from build123d import *

# Parameters (mm, degrees)
SKETCH1_W          = 34
SKETCH1_H          = 25
EXTRUDE1_DEPTH     = 30
SKETCH2_W          = 34
SKETCH2_H          = 25
EXTRUDE2_DEPTH     = 5
CHAMFER1_SIZE      = 5
SKETCH3_R          = 1.75
CUT_EXTRUDE1_DEPTH = 47.717707411


with BuildPart() as part:
    # Sketch1 → Extrude1 (new body)
    with BuildSketch(Plane.XY):
        with Locations((-8.642624393, 54.051188485)):
            Rectangle(SKETCH1_W, SKETCH1_H)
    extrude(amount=-EXTRUDE1_DEPTH)

    # Sketch2 → Extrude2 (add)
    with BuildSketch(Plane.XY):
        with Locations((-8.642624393, 54.051188485)):
            Rectangle(SKETCH2_W, SKETCH2_H)
    extrude(amount=EXTRUDE2_DEPTH)

    # Chamfer1
    chamfer1_edges = [part.edges().sort_by_distance(p)[0] for p in [
        (8.357375607, 54.051188485, -30),
        (-25.642624393, 54.051188485, -30),
    ]]
    chamfer(chamfer1_edges, length=CHAMFER1_SIZE)

    # Sketch3 → Cut-Extrude1 (cut, through all)
    with BuildSketch(Plane.XZ.offset(-41.551188485)):
        with Locations((-16.392624393, -20)):
            Circle(SKETCH3_R)
        with Locations((-0.892624393, -20)):
            Circle(SKETCH3_R)
        with Locations((-20.642624393, -2)):
            Circle(SKETCH3_R)
        with Locations(Location((3.357375607, -2, 0), (0, 0, 180))):
            Circle(SKETCH3_R)
    extrude(amount=-CUT_EXTRUDE1_DEPTH, mode=Mode.SUBTRACT)


solid = part.part
Work out the finished part from the listing and answer in its coordinate system (mm). Give positions to 0.01 mm unless a question says otherwise; leave off trailing zeros. Loops run counter-clockwise (first coordinate to the right, second up) from the corner with the lowest first, then second, coordinate; pieces in that order, holes last. Notation, with made-up numbers: (69.5, 8) -> (88.5, 8) arc R22 ccw to (88.5, 16) -> close; hole circle Ø3 at (55.25, 58.25). An arc over 180 degrees is marked (long way). Use a Markdown table: item, result. Add a question column.
1) The part is cut by section C-C, the plane x = 4.5. Determine the outline of the cut face in (y, z).
2) For a pull along X with two mould halves and no side action, classify faces 1 (the cylindrical face through (-16.62, 53.876, -18.265)), 2 (the cylindrical face through (3.737, 53.876, -0.292)), 3 (the flat face through (-25.643, 54, -10)), 4 (the flat face through (-9, 54, -30)) as +X half, -X half, draft (parallel to the pull), parting line (faces both ways), or undercut.
3) Consider line 1 along X through (y, z) = (51.75, -19.5); line 2 along Z through (x, y) = (-2, 64.75); line 3 along Z through (x, y) = (4, 61). Determine where each line is inside the solid, lowest interval first.
4) The part is cut by section B-B, the plane y = 48. Determine the outline of the cut face in (x, z).
5) The part is cut by section A-A, the plane z = -20. Determine the outline of the cut face in (x, y).
Reported:
| question | item | result |
|---|---|---|
| 1 | outline | (41.55, -28.86) -> (66.55, -28.86) -> (66.55, -3.33) -> (41.55, -3.33) -> close; (41.55, -0.67) -> (66.55, -0.67) -> (66.55, 5) -> (41.55, 5) -> close |
| 2 | face 1 | undercut |
| 2 | face 2 | undercut |
| 2 | face 3 | -X half |
| 2 | face 4 | draft |
| 3 | line 1 | x = -25.64 to -18.07, -14.72 to -2.57, 0.78 to 8.36 |
| 3 | line 2 | z = -30 to -21.36, -18.64 to 5 |
| 3 | line 3 | z = -29.36 to -3.63, -0.37 to 5 |
| 4 | outline | (-25.64, -25) -> (-20.64, -30) -> (3.36, -30) -> (8.36, -25) -> (8.36, 5) -> (-25.64, 5) -> close; hole circle Ø3.5 at (-20.64, -2); hole circle Ø3.5 at (-16.39, -20); hole circle Ø3.5 at (-0.89, -20); hole circle Ø3.5 at (3.36, -2) |
| 5 | outline | (-25.64, 41.55) -> (-18.14, 41.55) -> (-18.14, 66.55) -> (-25.64, 66.55) -> close; (-14.64, 41.55) -> (-2.64, 41.55) -> (-2.64, 66.55) -> (-14.64, 66.55) -> close; (0.86, 41.55) -> (8.36, 41.55) -> (8.36, 66.55) -> (0.86, 66.55) -> close |
